Autodesk Inventor part; units mm, degrees
ref_plane "YZ Plane" through (0, 0, 0) normal (1, 0, 0) x (0, 1, 0)
ref_plane "XZ Plane" through (0, 0, 0) normal (0, 1, 0) x (-1, 0, 0)
ref_plane "XY Plane" through (0, 0, 0) normal (0, 0, 1) x (1, 0, 0)
sketch "Sketch1" plane through (0, 0, 0) normal (0, 1, 0) x (-1, 0, 0)
  circle A0 centre (0, 0) radius 8
  dimension "d0" = 16
extrude "Extrusion1" add sketch "Sketch1" along normal blind 0.01
sketch "Sketch2" plane through (0, 0.01, 0) normal (0, 1, 0) x (1, 0, 0)
  circle A0 centre (0, 0) radius 6
  dimension "d3" = 12
extrude "Extrusion2" add sketch "Sketch2" along normal blind 8.5
sketch "Sketch3" plane through (0, 8.51, 0) normal (0, 1, 0) x (1, 0, 0)
  circle A0 centre (0, 0) radius 6
  line L0 (0, -6) -> (0, 6)
  line L1 (-6, 0) -> (6, 0)
hole "Hole1" at (0, 8.51, 0) direction (0, -1, 0) diameter 10 end through all
properties part number "Drukhulse ff"
Geometry check sheet. Reference: the model listing, model coordinates, mm. A direction names the side the tool comes from. Round coordinates to 2 decimals unless told otherwise and drop trailing zeros. Order: outer loops, then holes, each group sorted by start corner. A loop starts at its lowest first (then second) coordinate and runs counter-clockwise, first axis right, second up. Notation, with made-up numbers: (68, 34.5) - (74, 34.5) arc R21 cw to (74, 65.5) - close; hole circle Ø2 at (-2.5, 3). An arc over 180 degrees is marked (long way). Use a Markdown table: item, result. Add a question column.
(1) Depth check by flat-ended pin: pin 1 (5 mm diameter, centred on x = -4.5, y = 3, fed in from -Z); pin 2 (4 mm diameter, centred on x = -1, z = -2.5, fed in from -Y); pin 3 (2 mm diameter, centred on y = 5.5, z = 2, fed in from +X); pin 4 (5 mm diameter, centred on y = 3, z = 3, fed in from +X). Enter the tip coordinate at first touch or a pass-through.
(2) Material ranges on line 1 along Z through (x, y) = (0, 5); line 2 along X through (y, z) = (3, -1.5), recorded low to high. Write a range as [from, to].
(3) Sectioned sample at C-C, the plane y = 2.25. Enter the section's corners in (x, z), and give its area (3 significant figures).
(4) Tool access check on faces 1 (the flat face through (0.1, 0, -5.2)), 2 (the cylindrical face through (-6, 4, 0)). Record the directions out of +Z, -Z, +X, -X, +Y, -Y that give a thin tool (end or side, any length) a straight path to the whole face; none if there is none.
Answers below:
| question | item | result |
|---|---|---|
| 1 | pin 1 | z = -5.66 |
| 1 | pin 2 | through |
| 1 | pin 3 | x = 5.92 |
| 1 | pin 4 | x = 5.98 |
| 2 | line 1 | [-6, -5], [5, 6] |
| 2 | line 2 | [-5.81, -4.77], [4.77, 5.81] |
| 3 | outline | circle Ø12 at (0, 0); hole circle Ø10 at (0, 0) |
| 3 | area | 34.6 mm² |
| 4 | face 1 | +Z, -Z, +X, -X, -Y |
| 4 | face 2 | +Y |
